Autodesk Inventor part; units mm, degrees
ref_plane "YZ Plane" through (0, 0, 0) normal (1, 0, 0) x (0, 1, 0)
ref_plane "XZ Plane" through (0, 0, 0) normal (0, 1, 0) x (-1, 0, 0)
ref_plane "XY Plane" through (0, 0, 0) normal (0, 0, 1) x (1, 0, 0)
sketch "Sketch1" plane through (0, 0, 0) normal (0, 1, 0) x (-1, 0, 0)
  line L0 (0, 0) -> (88.25, 0)
  line L1 (88.25, 0) -> (88.25, -30)
  line L2 (88.25, -30) -> (0, -30)
  line L3 (0, -30) -> (0, 0)
  dimension "d0" = 88.25
  dimension "d1" = 30
extrude "Extrusion1" add sketch "Sketch1" along normal blind 2
sketch "Sketch2" plane through (0, 2, 0) normal (0, 1, 0) x (1, 0, 0)
  line L0 (-11.2333, 0) -> (-11.2333, 30)
  line L1 (0, 30) -> (-88.25, 30)
  line L2 (-16.7102, 0) -> (-16.7102, 3)
  line L3 (-16.7102, 30) -> (-16.7102, 27)
  line L4 (-16.7102, 3) -> (-16.7102, 5.125)
  circle A0 centre (-16.7102, 5.125) radius 2.125
  line L5 (-16.7102, 15) -> (-76.7102, 15)
  line L6 (-76.7102, 27) -> (-84.8352, 27)
  line L7 (-16.7102, 22.536) -> (-8.5852, 22.536)
  line L8 (-84.8352, 30) -> (-88.25, 30)
  line L9 (-88.25, 30) -> (-88.25, 0)
  line L10 (-88.25, 0) -> (-84.8352, 0)
  line L11 (-84.8352, 0) -> (-84.8352, 30)
  line L12 (-8.5852, 0) -> (0, 0)
  line L13 (0, 0) -> (0, 30)
  line L14 (0, 30) -> (-8.5852, 30)
  line L15 (-8.5852, 30) -> (-8.5852, 0)
  dimension "d4" = 3
  dimension "d5" = 3
  dimension "d6" = 30
  dimension "d7" = 2.125
  dimension "d8" = 4.25
  dimension "d9" = 60
  dimension "d12" = 8.125
  dimension "d13" = 8.125
extrude "Extrusion2" cut sketch "Sketch2" against normal through all contours A0
pattern_linear "Rectangular Pattern1" count 6 spacing 12 along (-1, 0, 0) count 2 spacing 18 along (0, 0, -1) of "Extrusion2"
sketch "Sketch3" plane through (0, 2, 0) normal (0, 1, 0) x (1, 0, 0)
  line L0 (0, 30) -> (0, 0)
  line L1 (-88.25, 0) -> (0, 0)
  line L2 (0, 0) -> (0, 2)
  line L3 (0, 2) -> (-88.25, 2)
  line L4 (-88.25, 2) -> (-88.25, 0)
  line L5 (0, 0) -> (0, 30)
  line L6 (-88.25, 30) -> (0, 30)
  line L7 (0, 30) -> (0, 28)
  line L8 (0, 28) -> (-88.25, 28)
  line L9 (-88.25, 28) -> (-88.25, 30)
  dimension "d22" = 2
  dimension "d23" = 2
extrude "Extrusion3" add sketch "Sketch3" along normal blind 26
sketch "Sketch4" plane through (-88.25, 0, 0) normal (0, 0, 1) x (1, 0, 0)
  line L0 (88.25, 28) -> (0.1331, 28)
  line L1 (0.1331, 28) -> (0.1331, 30)
  line L2 (0.1331, 30) -> (88.25, 30)
  line L3 (88.25, 30) -> (88.25, 28)
  point P0 (88.25, 0)
  dimension "d26" = 2
extrude "Extrusion4" add sketch "Sketch4" against normal blind 30
sketch "Sketch5" plane through (-88.1169, 30, 0) normal (0, 1, 0) x (1, 0, 0)
  circle A0 centre (71.4066, 5.125) radius 2.125
  circle A1 centre (71.4066, 5.125) radius 2.125
  point P0 (88.1169, 0)
extrude "Extrusion5" cut sketch "Sketch5" against normal through all
pattern_linear "Rectangular Pattern2" count 6 spacing 12 along (-1, 0, 0) count 2 spacing 18 along (0, 0, -1) of "Extrusion5"
sketch "Sketch6" plane through (0, 0, -30) normal (0, 0, -1) x (-1, 0, 0)
  line L0 (18.8352, 0) -> (14.5852, 0)
  circle A0 centre (16.7102, 6.1249) radius 2.125
  point P0 (0, 0)
  dimension "d37" = 4.25
extrude "Extrusion6" cut sketch "Sketch6" against normal through all
pattern_linear "Rectangular Pattern3" count 6 spacing 12 along (-1, 0, 0) count 2 spacing 18 along (0, 1, 0) of "Extrusion6"
equation "\"d38\" = d37"
properties part number "BatHoldV2"
Geometry check sheet. Reference: the model listing, model coordinates, mm. A direction names the side the tool comes from. Round coordinates to 2 decimals unless told otherwise and drop trailing zeros. Order: outer loops, then holes, each group sorted by start corner. A loop starts at its lowest first (then second) coordinate and runs counter-clockwise, first axis right, second up. Notation, with made-up numbers: M 36.25,25.5 L 85.25,25.5 A8 cw 85.25,40.5 Z; hole C -39.75,35 d11. An arc over 180 degrees is marked long. Answer in a Markdown table with one row per item.
(1) Sectioned sample at B-B, the plane z = -19.75. Record the cut outline in (x, y).
Responses:
| item | result |
|---|---|
| outline | M -88.25,0 L 0,0 L 0,2 L -88.25,2 Z; M -88.12,28 L 0,28 L 0,30 L -88.12,30 Z |
(2) Draft check along X on faces 3 (the face through (-45, 15, 0)), 4 (the face through (-88.25, 1, -13)), 5 (the face through (-50.587, 24.218, -29.014)). Enter one of: released by +X, released by -X, zero draft, split by the parting line, or undercut.
Responses:
| item | result |
|---|---|
| face 3 | zero draft |
| face 4 | released by -X |
| face 5 | undercut |
(3) Go/stop test with a flat-tipped pin: P1, Ø3.5, axis at x = -52.71, y = 24.12, coming from the -Z side. Record where the tip stops, or that it passes through.
Responses:
| item | result |
|---|---|
| P1 | passes through |
(4) Scan lines: probe 1 along Z at (x, y) = (-84, 11.75); probe 2 along Y at (x, z) = (-60.5, -8.25); probe 3 along Y at (x, z) = (-63, -28.5). Record each from-to range of solid material in increasing order. Write a range as from..to.
Responses:
| item | result |
|---|---|
| probe 1 | z = -30..-28, -2..0 |
| probe 2 | y = 0..2, 28..30 |
| probe 3 | y = 0..4.86, 7.39..22.86, 25.39..30 |
(5) Sectioned sample at C-C, the plane x = -20. Record the cut outline in (y, z), and give its area (3 significant figures).
Responses:
| item | result |
|---|---|
| outline | M 0,-30 L 30,-30 L 30,0 L 0,0 Z; hole M 2,-28 L 28,-28 L 28,-2 L 2,-2 Z |
| area | 224 mm² |
(6) Sectioned sample at A-A, the plane y = 19.75. Record the cut outline in (x, z), and give its area (3 significant figures).
Responses:
| item | result |
|---|---|
| outline | M -88.25,-30 L 0,-30 L 0,-28 L -88.25,-28 Z; M -88.25,-2 L 0,-2 L 0,0 L -88.25,0 Z |
| area | 353 mm² |
(7) Tool access check on faces 1 (the face through (-50.587, 24.218, -1.014)), 2 (the face through (-44, 15, -2)). Record the directions out of +Z, -Z, +X, -X, +Y, -Y that give a thin tool (end or side, any length) a straight path to the whole face; none if there is none.
Responses:
| item | result |
|---|---|
| face 1 | +Z, -Z |
| face 2 | +X, -X |
(8) Sectioned sample at D-D, the plane z = -4.25. State how many separate pieces and enclosed holes the cut face has, and give its area (3 significant figures).
Responses:
| item | result |
|---|---|
| separate pieces | 14 |
| enclosed holes | 0 |
| area | 260 mm² |
